The listing builds one solid part. Answer for the finished solid, in the listing's coordinates (mm). A direction names the side the tool comes from. Coordinates: 2 decimals unless noted, no trailing zeros. Order: outer loops, then holes, each group sorted by start corner. A loop starts at its lowest first (then second) coordinate and runs counter-clockwise, first axis right, second up. Notation, with made-up numbers: (6.5, 86) - (33.5, 86) arc R28 ccw to (33.5, 117) - close; hole circle Ø11 at (-26, 88). An arc over 180 degrees is marked (long way). Use a Markdown table: item, result. Add a question column.
Item 1: For faces 1 (the flat face through (5, 40, 11)), 2 (the flat face through (10, 22, 7)), 3 (the flat face through (5, 16, 3.5)), determine the directions among +Z, -Z, +X, -X, +Y, -Y from which every point of the face is accessible in a straight line to the end or side of a thin tool.
Item 2: The part is cut by section C-C, the plane z = 5. Give the vertices of the cut face in (x, y).
Item 3: The part is cut by section A-A, the plane y = 25. Give the vertices of the cut face in (x, z), then the cut area to 3 significant figures.
Item 4: Find the intervals of material crossed by line 1 along Z through (x, y) = (7, 17); line 2 along Y through (x, z) = (6.5, 12.5); line 3 along Y through (x, z) = (8, 6.25), in increasing order.
Item 5: The part is cut by section B-B, the plane x = 1. Give the vertices of the cut face in (y, z), then the cut area to 3 significant figures.
Item 6: The mould has two halves that part along Z. Classify faces 4 (the flat face through (5, 23, -5)), 5 (the flat face through (5, 38, 15.3)), 6 (the flat face through (5, 23, 20)), 7 (the flat face through (5, 36.5, 11)): released by +Z, released by -Z, zero draft, split by the parting line, or undercut.
from build123d import *

# Parameters (mm, degrees)
BOX_W        = 10
BOX_H        = 45
BOX_DEPTH    = 25
POCKET_DEPTH = 10


with BuildPart() as part:
    # Box → Box (join)
    with BuildSketch(Plane.XY.offset(-5)):
        with Locations((5, 22.5)):
            Rectangle(BOX_W, BOX_H)
    extrude(amount=BOX_DEPTH)

    # Sketch → Pocket (cut)
    with BuildSketch(Plane.YZ):
        with BuildLine():
            Line((40, 15.3), (40, 6))
            ThreePointArc((34, 0), (38.242641, 1.757359), (40, 6))
            Line((0, 0), (34, 0))
            Line((0, 3.5), (0, 0))
            Line((32.5, 3.5), (0, 3.5))
            ThreePointArc((32.5, 3.5), (35.328427, 4.671573), (36.5, 7.5))
            Line((36.5, 15.3), (36.5, 7.5))
            Line((36.5, 15.3), (40, 15.3))
        make_face()
    extrude(amount=POCKET_DEPTH, mode=Mode.SUBTRACT)


solid = part.part
Solution:
| question | item | result |
|---|---|---|
| 1 | face 1 | +X, -X |
| 1 | face 2 | +Z, -Z, +X, +Y, -Y |
| 1 | face 3 | +X, -X, -Y |
| 2 | outline | (0, 0) - (10, 0) - (10, 35.62) - (0, 35.62) - close; (0, 39.92) - (10, 39.92) - (10, 45) - (0, 45) - close |
| 3 | outline | (0, -5) - (10, -5) - (10, 0) - (0, 0) - close; (0, 3.5) - (10, 3.5) - (10, 20) - (0, 20) - close |
| 3 | area | 215 mm2 |
| 4 | line 1 | z = -5 to 0, 3.5 to 20 |
| 4 | line 2 | y = 0 to 36.5, 40 to 45 |
| 4 | line 3 | y = 0 to 36.3, 40 to 45 |
| 5 | outline | (0, -5) - (45, -5) - (45, 20) - (0, 20) - (0, 3.5) - (32.5, 3.5) arc R4 ccw to (36.5, 7.5) - (36.5, 15.3) - (40, 15.3) - (40, 6) arc R6 cw to (34, 0) - (0, 0) - close |
| 5 | area | 948 mm2 |
| 6 | face 4 | released by -Z |
| 6 | face 5 | undercut |
| 6 | face 6 | released by +Z |
| 6 | face 7 | undercut |
